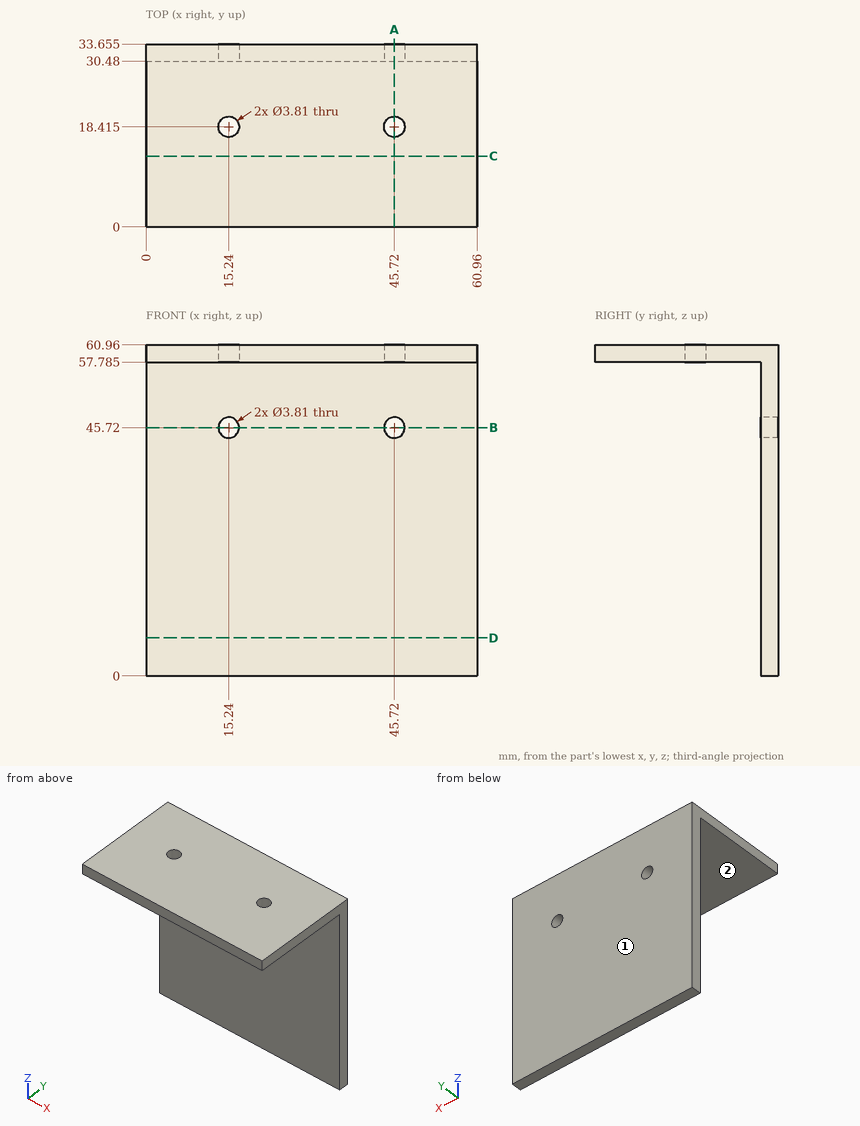
Could you check a few things on this drawing? It's one solid part, dimensions in mm from its lowest x, y, z. A direction names the side the tool comes from. Round coordinates to 2 decimals unless told otherwise and drop trailing zeros. Write each loop counter-clockwise with the first axis right and the second up, starting at its lowest first coordinate (ties: lowest second). Pieces come first, ordered by that corner, then holes.
Q1. If we section it at B-B on z = 45.72: Write out the boundary of the cut face in (x, y) (3 decimals), plus the area to 3 significant figures.
Q2. If we section it at D-D on z = 7: Write out the boundary of the cut face in (x, y) (3 decimals), plus the area to 3 significant figures.
Q3. Which directions (+Z, -Z, +X, -X, +Y, -Y) give clear straight access to the entire face, cutting with the end or side of a thin tool? Please do the marked faces 1 and 2.
Q4. If we section it at A-A on x = 45.72: Write out the boundary of the cut face in (y, z) (3 decimals), plus the area to 3 significant figures.
Q5. Will these pins go through, and if not, where does the flat tip stop? P1, Ø9, axis at x = 28.5, y = 22.5, coming from the -Z side (3 decimals); P2, Ø1.5, axis at x = 33, z = 50, coming from the -Y side.
Q6. Please list where these lines run through material, in increasing order: probe 1 along X at (y, z) = (32.05, 45.72) (3 decimals); probe 2 along Y at (x, z) = (15, 58) (3 decimals); probe 3 along X at (y, z) = (31, 45).
Q7. If we section it at C-C on y = 13: Write out the boundary of the cut face in (x, z) (3 decimals).
Answer below:
1. outline: (0, 30.48) - (13.335, 30.48) - (13.335, 33.655) - (0, 33.655) - close; (17.145, 30.48) - (43.815, 30.48) - (43.815, 33.655) - (17.145, 33.655) - close; (47.625, 30.48) - (60.96, 30.48) - (60.96, 33.655) - (47.625, 33.655) - close
1. area: 169 mm2
2. outline: (0, 30.48) - (60.96, 30.48) - (60.96, 33.655) - (0, 33.655) - close
2. area: 194 mm2
3. face 1: +Z, -Z, +X, -X, +Y
3. face 2: -Z, +X, -X, -Y
4. outline: (0, 57.785) - (16.51, 57.785) - (16.51, 60.96) - (0, 60.96) - close; (20.32, 57.785) - (30.48, 57.785) - (30.48, 47.625) - (33.655, 47.625) - (33.655, 60.96) - (20.32, 60.96) - close; (30.48, 0) - (33.655, 0) - (33.655, 43.815) - (30.48, 43.815) - close
4. area: 266 mm2
5. P1: stops at z = 57.785
5. P2: stops at y = 30.48
6. probe 1: x = 0 to 13.335, 17.145 to 43.815, 47.625 to 60.96
6. probe 2: y = 0 to 16.525, 20.305 to 33.655
6. probe 3: x = 0 to 13.48, 17 to 43.96, 47.48 to 60.96
7. outline: (0, 57.785) - (60.96, 57.785) - (60.96, 60.96) - (0, 60.96) - close
